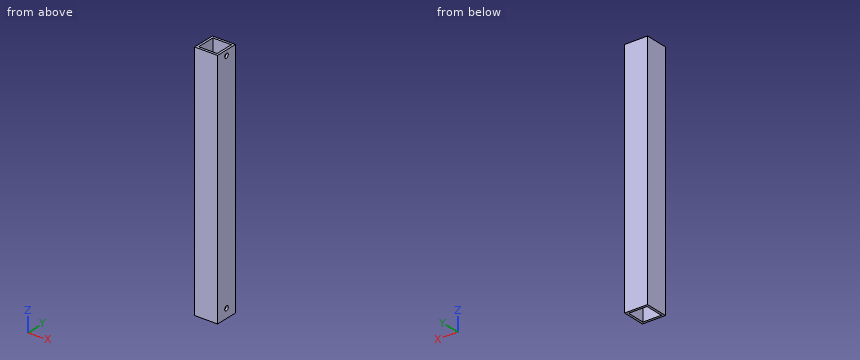
Autodesk Inventor part; units mm, degrees
ref_plane "YZ Plane" through (0, 0, 0) normal (1, 0, 0) x (0, 1, 0)
ref_plane "XZ Plane" through (0, 0, 0) normal (0, 1, 0) x (-1, 0, 0)
ref_plane "XY Plane" through (0, 0, 0) normal (0, 0, 1) x (1, 0, 0)
sketch "Sketch1" plane through (0, 0, 0) normal (0, 0, 1) x (1, 0, 0)
  line L0 (12.7, -12.7) -> (-12.7, -12.7)
  line L1 (-12.7, -12.7) -> (-12.7, 12.7)
  line L2 (-12.7, 12.7) -> (12.7, 12.7)
  line L3 (12.7, 12.7) -> (12.7, -12.7)
  line L4 (12.7, -12.7) -> (-12.7, 12.7) construction
  line L5 (-12.7, -12.7) -> (12.7, 12.7) construction
  line L6 (10.16, 10.16) -> (-10.16, 10.16)
  line L7 (-10.16, 10.16) -> (-10.16, -10.16)
  line L8 (-10.16, -10.16) -> (10.16, -10.16)
  line L9 (10.16, -10.16) -> (10.16, 10.16)
  line L10 (10.16, 10.16) -> (-10.16, -10.16) construction
  line L11 (-10.16, 10.16) -> (10.16, -10.16) construction
  point P0 (0, 0)
  dimension "d0" = 25.4
  dimension "d1" = 25.4
  dimension "d2" = 2.54
  dimension "d3" = 2.54
extrude "Extrusion1" add sketch "Sketch1" along normal blind 266.7
sketch "Sketch2" plane through (12.7, -12.7, 0) normal (1, 0, 0) x (0, 0, -1)
  circle A0 centre (-10.1228, 12.7) radius 2.54
  circle A1 centre (-261.024, 12.7) radius 2.54
  line L0 (0, 25.4) -> (0, 0)
  line L1 (-266.7, 0) -> (-266.7, 25.4)
  line L2 (0, 0) -> (-266.7, 0)
  point P0 (0, 12.7)
  dimension "d6" = 250.9012
  dimension "d7" = 5.08
  dimension "d8" = 5.08
  dimension "d15" = 12.7
  dimension "d16" = 12.7
extrude "Extrusion2" cut sketch "Sketch2" against normal blind 2.54
equation "\"d3\" = d2"
equation "\"d8\" = d7"
properties part number "push bar"
Could you check a few things on this model? Use its own coordinates, in mm. Coordinates: 2 decimals unless noted, no trailing zeros. Loops run counter-clockwise (first coordinate to the right, second up) from the corner with the lowest first, then second, coordinate; pieces in that order, holes last. Notation, with made-up numbers: (71, 65.25) -> (89, 65.25) arc R12 cw to (89, 74.25) -> close; hole circle Ø5 at (57, 78). An arc over 180 degrees is marked (long way). Answer in a Markdown table with one row per item.
(1) Imagine slicing it at C-C (z = 45). List the corners of the cut face in (x, y) for me.
Results found:
| item | result |
|---|---|
| outline | (-12.7, -12.7) -> (12.7, -12.7) -> (12.7, 12.7) -> (-12.7, 12.7) -> close; hole (-10.16, -10.16) -> (10.16, -10.16) -> (10.16, 10.16) -> (-10.16, 10.16) -> close |
(2) Imagine slicing it at B-B (x = 4.25). List the corners of the cut face in (y, z) for me, plus the area to 3 significant figures.
Results found:
| item | result |
|---|---|
| outline | (-12.7, 0) -> (-10.16, 0) -> (-10.16, 266.7) -> (-12.7, 266.7) -> close; (10.16, 0) -> (12.7, 0) -> (12.7, 266.7) -> (10.16, 266.7) -> close |
| area | 1,350 mm^2 |
(3) Imagine slicing it at A-A (y = 0). List the corners of the cut face in (x, z) for me, plus the area to 3 significant figures.
Results found:
| item | result |
|---|---|
| outline | (-12.7, 0) -> (-10.16, 0) -> (-10.16, 266.7) -> (-12.7, 266.7) -> close; (10.16, 0) -> (12.7, 0) -> (12.7, 7.58) -> (10.16, 7.58) -> close; (10.16, 12.66) -> (12.7, 12.66) -> (12.7, 258.48) -> (10.16, 258.48) -> close; (10.16, 263.56) -> (12.7, 263.56) -> (12.7, 266.7) -> (10.16, 266.7) -> close |
| area | 1,330 mm^2 |
(4) If I drill on probe 1 along X at (y, z) = (8.25, 139.5); probe 2 along Z at (x, y) = (11.5, -1.25), over which ranges is the centre line in solid material (lowest first)?
Results found:
| item | result |
|---|---|
| probe 1 | x = -12.7 to -10.16, 10.16 to 12.7 |
| probe 2 | z = 0 to 7.91, 12.33 to 258.81, 263.24 to 266.7 |
